Geometry check sheet. Reference: the model listing, model coordinates, mm. A direction names the side the tool comes from. Coordinates: 2 decimals unless noted, no trailing zeros. Write each loop counter-clockwise with the first axis right and the second up, starting at its lowest first coordinate (ties: lowest second). Pieces come first, ordered by that corner, then holes. Notation, with made-up numbers: (42, 24.25) -> (77, 24.25) arc R13 ccw to (77, 47.25) -> close; hole circle Ø7 at (-17, -21). An arc over 180 degrees is marked (long way). Answer as CSV lines item,"result".
Autodesk Fusion 360 part; units mm, degrees
sketch "Sketch1" plane through (0, 0, 0) normal (0, 0, 1) x (1, 0, 0)
  line L0 (0, 0) -> (60.88, 0)
  line L1 (60.88, 0) -> (60.88, 108)
  line L2 (60.88, 108) -> (0, 108)
  line L3 (0, 108) -> (0, 0)
  circle A0 centre (3, 3) radius 1.6
  circle A1 centre (57.88, 3) radius 1.6
  circle A2 centre (3, 105) radius 1.6
  circle A3 centre (57.88, 105) radius 1.6
  line L4 (0, 101.29) -> (60.88, 101.29)
  line L5 (60.88, 101.29) -> (60.88, 6.72)
  line L6 (60.88, 6.72) -> (0, 6.72)
  line L7 (0, 6.72) -> (0, 101.29)
  dimension "d1" = 60.88
  dimension "d2" = 108
  dimension "d3" = 3.2
  dimension "d6" = 54.88
  dimension "d7" = 102
  dimension "d8" = 3
  dimension "d9" = 3
  dimension "d10" = 60.88
  dimension "d11" = 94.57
  dimension "d12" = 6.71
extrude "Extrude1" add sketch "Sketch1" along normal blind 1.6 contours L0 L1 L3 L6 | L1 L2 L3 L4 makes body 1 at (39.32, 102.0648, 0) makes body 2 at (21.56, 5.9419, 0)
extrude "Extrude2" add sketch "Sketch1" along normal blind 6.45 contours L1 L3 L4 L5 L6 L7 bodies 1 2
sketch "Sketch2" plane through (0, 0, 0) normal (0, 0, -1) x (1, 0, 0)
  circle A0 centre (57.88, -3) radius 1.6
  circle A1 centre (3, -3) radius 1.6
  circle A2 centre (57.88, -105) radius 1.6
  circle A3 centre (3, -105) radius 1.6
  line L0 (0, 0) -> (0, -108)
  line L1 (0, -108) -> (60.88, -108)
  line L2 (60.88, -108) -> (60.88, 0)
  line L3 (60.88, 0) -> (0, 0)
  line L4 (17, -63.47) -> (0, -63.47)
  line L5 (0, -63.47) -> (0, -48.47)
  line L6 (0, -48.47) -> (17, -48.47)
  line L7 (17, -48.47) -> (17, -63.47)
  point P0 (0, -55.97)
  dimension "d18" = 17
  dimension "d19" = 15
  dimension "d20" = 52.03
extrude "Extrude3" add sketch "Sketch2" along normal blind 2.2 contours L0 L4 L5 L6 L7 bodies 1
sketch "Sketch3" plane through (0, 0, 1.6) normal (0, 0, 1) x (-1, 0, 0)
  circle A0 centre (-3, -3) radius 1.6
  circle A1 centre (-57.88, -3) radius 1.6
  line L0 (-60.88, -6.72) -> (0, -6.72)
  line L1 (0, -6.72) -> (0, 0)
  line L2 (0, 0) -> (-60.88, 0)
  line L3 (-60.88, 0) -> (-60.88, -6.72)
  line L4 (-12.94, -3.27) -> (-47.94, -3.27)
  line L5 (-47.94, -3.27) -> (-47.94, -0.73)
  line L6 (-47.94, -0.73) -> (-12.94, -0.73)
  line L7 (-12.94, -0.73) -> (-12.94, -3.27)
  point P0 (-30.44, -3.27)
  point P1 (-47.94, -2)
  point P2 (-30.44, 0)
  point P3 (-30.44, -0.73)
  dimension "d23" = 35
  dimension "d24" = 2.54
  dimension "d25" = 2
extrude "Extrude4" add sketch "Sketch3" along normal blind 1.23 and the other way blind 9.94 contours L4 L5 L6 L7 bodies 1
equation "d28 = 11.17 mm - 1.23 mm"
Item 1: Cross-section at A-A, the plane y = 105. Record the cut outline in (x, z), plus the area to 3 significant figures.
Responses:
outline,"(0, 0) -> (1.4, 0) -> (1.4, 1.6) -> (0, 1.6) -> close; (4.6, 0) -> (56.28, 0) -> (56.28, 1.6) -> (4.6, 1.6) -> close; (59.48, 0) -> (60.88, 0) -> (60.88, 1.6) -> (59.48, 1.6) -> close"
area,"87.2 mm2"
Item 2: Release check for a two-part mould opening along X. For faces 4 (the flat face through (31, 2, 2.83)), 5 (the cylindrical face through (1.73, 3.97, 0.79)), 6 (the cylindrical face through (59.4, 104.5, 0.8)), 7 (the flat face through (17, 56, -1)) record: +X half, -X half, draft (parallel to the pull), parting line (faces both ways), or undercut.
Responses:
face 4,"draft"
face 5,"undercut"
face 6,"undercut"
face 7,"+X half"
Item 3: Cross-section at B-B, the plane x = 57.88. Record the cut outline in (y, z).
Responses:
outline,"(0, 0) -> (1.4, 0) -> (1.4, 1.6) -> (0, 1.6) -> close; (4.6, 0) -> (103.4, 0) -> (103.4, 1.6) -> (101.29, 1.6) -> (101.29, 6.45) -> (6.72, 6.45) -> (6.72, 1.6) -> (4.6, 1.6) -> close; (106.6, 0) -> (108, 0) -> (108, 1.6) -> (106.6, 1.6) -> close"
Item 4: Cross-section at D-D, the plane z = -4.5. Record the cut outline in (x, y), plus the area to 3 significant figures.
Responses:
outline,"(12.94, 0.73) -> (47.94, 0.73) -> (47.94, 3.27) -> (12.94, 3.27) -> close"
area,"88.9 mm2"
Item 5: Thickness scan on probe 1 along Y at (x, z) = (3, 0.4); probe 2 along X at (y, z) = (105, 0.4); probe 3 along Z at (x, y) = (17, 29). Record the ranges inside material, lowest first.
Responses:
probe 1,"y = 0 to 1.4, 4.6 to 103.4, 106.6 to 108"
probe 2,"x = 0 to 1.4, 4.6 to 56.28, 59.48 to 60.88"
probe 3,"z = 0 to 6.45"
Item 6: Set-up check for faces 1 (the flat face through (31, 0.73, -4)), 2 (the flat face through (8, 56, -2.2)), 3 (the flat face through (30, 101.29, 4)): record each of +Z, -Z, +X, -X, +Y, -Y from which the full face is reachable in a straight line by a thin tool's end or side.
Responses:
face 1,"-Z, +X, -X, -Y"
face 2,"-Z, +X, -X, +Y"
face 3,"+Z, +X, -X, +Y"
Item 7: Cross-section at C-C, the plane x = 42. Record the cut outline in (y, z), plus the area to 3 significant figures.
Responses:
outline,"(0, 0) -> (0.73, 0) -> (0.73, -8.34) -> (3.27, -8.34) -> (3.27, 0) -> (108, 0) -> (108, 1.6) -> (101.29, 1.6) -> (101.29, 6.45) -> (6.72, 6.45) -> (6.72, 1.6) -> (3.27, 1.6) -> (3.27, 2.83) -> (0.73, 2.83) -> (0.73, 1.6) -> (0, 1.6) -> close"
area,"656 mm2"
Item 8: Depth check by flat-ended pin: pin 1 Ø3 at (x, y) = (39, 2) entering from +Z; pin 2 Ø1.8 at (x, z) = (11, -1) entering from -Y; pin 3 Ø0.8 at (y, z) = (1.5, -2.5) entering from -X. Enter the tip coordinate at first touch or a pass-through.
Responses:
pin 1,"stops at z = 2.83"
pin 2,"stops at y = 48.47"
pin 3,"stops at x = 12.94"
